Solid Edge part; units mm, degrees
sketch "Sketch1" plane through (0, 0, 0) normal (0, 0, 1) x (1, 0, 0)
  line L0 (-1.9657, 64.721) -> (-1.9657, 62.94)
  line L1 (-1.9657, 62.94) -> (-0.3373, 62.94)
  line L2 (-0.3373, 62.94) -> (-0.3373, 64.5683)
  line L3 (-0.3373, 64.5683) -> (1.291, 64.5683)
  line L4 (1.291, 64.5683) -> (0.9079, 66.1009)
  line L5 (0.9079, 66.1009) -> (-1.3239, 65.5429)
  line L6 (-1.3239, 65.5429) -> (-1.9657, 64.721)
revolve "RevolvedProtrusion1" add sketch "Sketch1" angle 360 about axis through (50, 0, 0) along (-1, 0, 0)
Here's how the part is built. I have some questions about the finished solid (model axes, mm). A direction names the side the tool comes from. Coordinates: 2 decimals unless noted, no trailing zeros. Write each loop counter-clockwise with the first axis right and the second up, starting at its lowest first coordinate (ties: lowest second). Pieces come first, ordered by that corner, then holes. Notation, with made-up numbers: M 37,10.5 L 41,10.5 A19 cw 41,31.5 Z; hole C -28.75,7.5 d1. An arc over 180 degrees is marked long. Answer as CSV lines item,"result". Start each with the question number.
Q1. Suppose I cut it at A-A, the plane y = 0. List the corners of the cut face in (x, z) for me.
Q2. I need wall thicknesses on probe 1 along Y at (x, z) = (0.8, 0); probe 2 along Z at (x, y) = (-1.2, 0); probe 3 along Y at (x, z) = (-0.6, -56). Which ranges of each line are inside material? Lowest first, please. Write a range as [from, to].
Q3. Will these pins go through, and if not, where does the flat tip stop? pin 1 Ø1.5 at (x, z) = (-0.5, 5) entering from -Y; pin 2 Ø1 at (x, z) = (-0.5, -50) entering from -Y.
Q4. If we mould it in two halves opening along Z, with no side actions, what happens to faces 1 (the flat face through (-1.966, 14, 62)), 2 (the flat face through (-0.337, 14, 62))? For each: pulls with the +Z half, pulls with the -Z half, needs draft (parallel to the pull), parting line crosses it, or undercut.
Q5. For faces 3 (the cylindrical face through (-1.14, -8.194, 62.404)), 4 (the cylindrical face through (0.49, -51.24, -39.29)), which set-ups out of +Z, -Z, +X, -X, +Y, -Y let a thin tool reach every point of the face, with its end or its side?
Entries:
1,outline,"M -1.97,-64.72 L -1.32,-65.54 L 0.91,-66.1 L 1.29,-64.57 L -0.34,-64.57 L -0.34,-62.94 L -1.97,-62.94 Z; M -1.97,62.94 L -0.34,62.94 L -0.34,64.57 L 1.29,64.57 L 0.91,66.1 L -1.32,65.54 L -1.97,64.72 Z"
2,probe 1,"y = [-66.07, -64.57], [64.57, 66.07]"
2,probe 2,"z = [-65.57, -62.94], [62.94, 65.57]"
2,probe 3,"y = [-34.4, -28.73], [28.73, 34.4]"
3,pin 1,"stops at y = -65.75"
3,pin 2,"stops at y = -43.31"
4,face 1,"needs draft"
4,face 2,"undercut"
5,face 3,"+X, -X"
5,face 4,"+X"
